Verification items for the finished model (mm, model axes). A direction names the side the tool comes from. Give positions to 0.01 mm unless a question says otherwise; leave off trailing zeros. Order: outer loops, then holes, each group sorted by start corner. A loop starts at its lowest first (then second) coordinate and runs counter-clockwise, first axis right, second up. Notation, with made-up numbers: (79.25, 64.5) -> (114.25, 64.5) arc R20 ccw to (114.25, 80.5) -> close; hole circle Ø11 at (-2.5, -1). An arc over 180 degrees is marked (long way). One line per question, with ' | ' between items. Start each with the question number.
Q1. Section check D-D on y = 22. Record the cut outline in (x, z).
Q2. Go/stop test with flat-tipped pins: pin 1 (5 mm diameter, centred on x = -15, z = 38, fed in from -Y); pin 2 (3 mm diameter, centred on y = 2, z = 49, fed in from -X); pin 3 (12 mm diameter, centred on x = 3.5, y = 10.5, fed in from -Z); pin 4 (1.5 mm diameter, centred on x = -2.5, z = 44, fed in from +Y). Record where each tip stops, or that it passes through.
Q3. Access from +Z, -Z, +X, -X, +Y, -Y to the whole of each face (thin tool, end or side, straight path). Record for faces 1 (the cylindrical face through (-5.234, -23.572, 42.325)), 2 (the flat face through (36.911, 0, 15)).
Q4. Section check B-B on y = 0. Record the cut outline in (x, z).
Q5. Section check A-A on x = 0. Record the cut outline in (y, z), plus the area to 3 significant figures.
Q6. Material ranges on probe 1 along Y at (x, z) = (0, 15.75); probe 2 along X at (y, z) = (-1, 24); probe 3 along Z at (x, y) = (6, 26.5), recorded low to high. Write a range as [from, to].
Q7. Section check C-C on z = 23.5. Record the cut outline in (x, y).
from build123d import *

# Parameters (mm, degrees)
F0_W     = 73.822246
F0_H     = 70.221156
F1_DEPTH = 30
F2_R     = 19.249212
F3_DEPTH = 30.001
F4_R     = 24.146454
F4_R_2   = 19.249212
F5_DEPTH = 25


with BuildPart() as f1:
    # F0 (on Top) → F1 (new body)
    with BuildSketch(Plane.XY):
        Rectangle(F0_W, F0_H)
    extrude(amount=F1_DEPTH)

    # F2 (on face) → F3 (cut, through all)
    with BuildSketch(Plane.XY.offset(30)):
        Circle(F2_R)
    extrude(amount=-F3_DEPTH, mode=Mode.SUBTRACT)

    # F4 (on face) → F5 (join)
    with BuildSketch(Plane.XY.offset(30)):
        Circle(F4_R)
        Circle(F4_R_2, mode=Mode.SUBTRACT)
    extrude(amount=F5_DEPTH)


solid = f1.part
Filled in:
1) outline: (-36.91, 0) -> (36.91, 0) -> (36.91, 30) -> (9.95, 30) -> (9.95, 55) -> (-9.95, 55) -> (-9.95, 30) -> (-36.91, 30) -> close
2) pin 1: y = -20.66 | pin 2: x = -24.14 | pin 3: through | pin 4: y = 24.08
3) face 1: +Z | face 2: +Z, -Z, +X, +Y, -Y
4) outline: (-36.91, 0) -> (-19.25, 0) -> (-19.25, 55) -> (-24.15, 55) -> (-24.15, 30) -> (-36.91, 30) -> close; (19.25, 0) -> (36.91, 0) -> (36.91, 30) -> (24.15, 30) -> (24.15, 55) -> (19.25, 55) -> close
5) outline: (-35.11, 0) -> (-19.25, 0) -> (-19.25, 55) -> (-24.15, 55) -> (-24.15, 30) -> (-35.11, 30) -> close; (19.25, 0) -> (35.11, 0) -> (35.11, 30) -> (24.15, 30) -> (24.15, 55) -> (19.25, 55) -> close | area: 1,200 mm²
6) probe 1: [-35.11, -19.25], [19.25, 35.11] | probe 2: [-36.91, -19.22], [19.22, 36.91] | probe 3: [0, 30]
7) outline: (-36.91, -35.11) -> (36.91, -35.11) -> (36.91, 35.11) -> (-36.91, 35.11) -> close; hole circle Ø38.5 at (0, 0)
